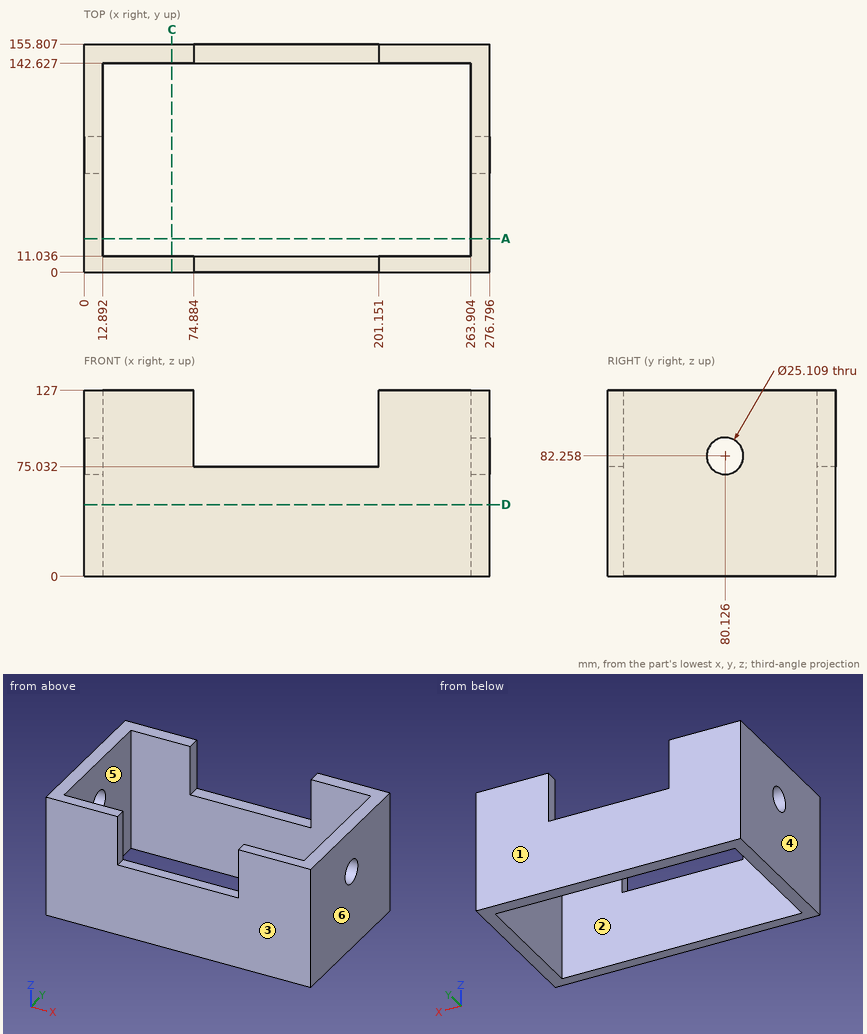
The drawing under review shows one solid part. Ordinate dimensions are in mm from its lowest x, y, z. A direction names the side the tool comes from. Coordinates: 2 decimals unless noted, no trailing zeros. Order: outer loops, then holes, each group sorted by start corner. A loop starts at its lowest first (then second) coordinate and runs counter-clockwise, first axis right, second up. Notation, with made-up numbers: (4.5, 12) - (25.5, 12) arc R27 ccw to (25.5, 42) - close; hole circle Ø9 at (-11, -37.5). An arc over 180 degrees is marked (long way). Put each result on its own line as item: value.
1) Wall thickness on L1, parallel to X at y = 23, z = 105.5 (1 decimal); L2, parallel to Y at x = 64.5, z = 22; L3, parallel to Z at x = 88, y = 146: over which ranges is each line inside the solid? List them lowest first. Write a range as from..to.
Response values:
L1: x = 0..12.9, 263.9..276.8
L2: y = 0..11.04, 142.63..155.81
L3: z = 0..75.03
2) The part is to be moulded in two halves that separate along Y. For the marked faces 1, 2, 3 and 4, say which applies: released by +Y, released by -Y, zero draft, split by the parting line, or undercut.
Response values:
face 1: released by +Y
face 2: undercut
face 3: released by -Y
face 4: zero draft
3) Take a section at D-D, the plane z = 49. Give the boundary of the cut face in (x, y) (1 decimal), and give its area (3 significant figures).
Response values:
outline: (0, 0) - (276.8, 0) - (276.8, 155.8) - (0, 155.8) - close; hole (12.9, 11) - (263.9, 11) - (263.9, 142.6) - (12.9, 142.6) - close
area: 10,100 mm²
4) Take a section at A-A, the plane y = 23. Give the boundary of the cut face in (x, z) (1 decimal).
Response values:
outline: (0, 0) - (12.9, 0) - (12.9, 127) - (0, 127) - close; (263.9, 0) - (276.8, 0) - (276.8, 127) - (263.9, 127) - close
5) Take a section at C-C, the plane x = 60. Give the boundary of the cut face in (y, z).
Response values:
outline: (0, 0) - (11.04, 0) - (11.04, 127) - (0, 127) - close; (142.63, 0) - (155.81, 0) - (155.81, 127) - (142.63, 127) - close
6) Insertion check: P1, Ø10.5, axis at x = 110, y = 151, coming from the +Z side. The pin has a flat end and moves straight along its axis. Give the tip position at first contact, or say it passes through.
Response values:
P1: stops at z = 75.03
7) Tool access review of the marked faces 5 and 6: name each direction out of +Z, -Z, +X, -X, +Y, -Y from which nothing blocks a thin tool from reaching the whole face with its end or side.
Response values:
face 5: +Z, -Z
face 6: +Z, -Z, +X, +Y, -Y
